Could you check a few things on this model? Use its own coordinates, in mm. A direction names the side the tool comes from. Give positions to 0.01 mm unless a question says otherwise; leave off trailing zeros. Loops run counter-clockwise (first coordinate to the right, second up) from the corner with the lowest first, then second, coordinate; pieces in that order, holes last. Notation, with made-up numbers: M -40,69 L -18,69 A10 ccw -18,75 Z; hole C -6,-14.5 d4. An arc over 180 degrees is marked long. Use a Markdown table: item, result. Add a question column.
1) If I drill on line 1 along Z through (x, y) = (3, 1.65); line 2 along Z through (x, y) = (11.2, 1.5); line 3 along Y through (x, z) = (4.5, 39) (3 decimals), over which ranges is the centre line in solid material (lowest first)? Write a range as [from, to].
2) Suppose I cut it at B-B on y = 0.75. List the corners of the cut face in (x, z) for me (3 decimals).
3) Suppose I cut it at A-A on x = 11.2. List the corners of the cut face in (y, z) for me (3 decimals).
4) Which directions (+Z, -Z, +X, -X, +Y, -Y) give clear straight access to the entire face, cutting with the end or side of a thin tool? Please do faces 4 (the cylindrical face through (1.098, 1.583, 33.354)), 5 (the flat face through (8, 1.905, 30)), 6 (the flat face through (15, 1.905, 30)).
5) Will these pins go through, and if not, where does the flat tip stop? pin 1 Ø0.7 at (x, z) = (1.5, 29) entering from +Y; pin 2 Ø2.5 at (x, z) = (3.5, 33) entering from +Y; pin 3 Ø0.9 at (x, z) = (22, 38) entering from +Y (3 decimals).
6) We'd pull the mould along X, two halves only. Please class faces 1 (the flat face through (20.196, 4.347, 30.128)), 2 (the flat face through (0, 1, 30)), 3 (the flat face through (1, 1.905, 30)): +X half, -X half, draft (parallel to the pull), parting line (faces both ways), or undercut.
```python
from build123d import *

# Parameters (mm, degrees)
SKETCH1_W               = 25.4
SKETCH1_H               = 1.905
BASE_DEPTH              = 61.1124
FINS_DEPTH              = 61.1124
CUT_EXTRUDE1_DEPTH      = 67.365786688
CUT_EXTRUDE1_DEPTH_BACK = 67.365786688
SKETCH3_R               = 1.9939


with BuildPart() as part:
    # Sketch1 → Base (new body)
    with BuildSketch(Plane.XY):
        with Locations((12.7, 0.9525)):
            Rectangle(SKETCH1_W, SKETCH1_H)
    extrude(amount=BASE_DEPTH)

    # Sketch2 → Fins (add)
    with BuildSketch(Plane(origin=(0, 0, 0), x_dir=(-1, 0, 0), z_dir=(0, 0, -1))):
        Polygon((-23.444268018, 1.905), (-25.4, 6.858), (-24.853831982, 6.858), (-22.8981, 1.905), align=None)
        Polygon((-20.040531982, 1.905), (-19.494363964, 1.905), (-20.916831982, 6.858), (-21.463, 6.858), align=None)
        Polygon((-16.979831982, 1.905), (-16.433663964, 1.905), (-16.979831982, 6.858), (-17.526, 6.858), align=None)
        Polygon((-2.794, 1.905), (-2.247831982, 1.905), (0, 6.858), (-0.546168018, 6.858), align=None)
        Polygon((-12.458768018, 6.858), (-11.9126, 6.858), (-12.598263964, 1.905), (-13.144431982, 1.905), align=None)
        Polygon((-8.216968018, 6.858), (-7.6708, 6.858), (-9.245463964, 1.905), (-9.791631982, 1.905), align=None)
        Polygon((-4.483168018, 6.858), (-3.937, 6.858), (-5.943463964, 1.905), (-6.489631982, 1.905), align=None)
    extrude(amount=-FINS_DEPTH)

    # Sketch3 → Cut-Extrude1 (cut, two sides: drawn at the far end of the back side and taken through both)
    with BuildSketch(Plane(origin=(0, 1.905, 0), x_dir=(1, 0, 0), z_dir=(0, 1, 0)).offset(-CUT_EXTRUDE1_DEPTH_BACK)):
        with Locations(Location((11.2, -9.655, 0), (0, 0, 180))):
            Circle(SKETCH3_R)
        with Locations(Location((3, -32.755, 0), (0, 0, 180))):
            Circle(SKETCH3_R)
    extrude(amount=CUT_EXTRUDE1_DEPTH + CUT_EXTRUDE1_DEPTH_BACK, mode=Mode.SUBTRACT)


solid = part.part
```
Answer block:
| question | item | result |
|---|---|---|
| 1 | line 1 | z = [0, 30.76], [34.75, 61.11] |
| 1 | line 2 | z = [0, 7.66], [11.65, 61.11] |
| 1 | line 3 | y = [0, 1.905], [5.468, 6.816] |
| 2 | outline | M 0,0 L 25.4,0 L 25.4,61.112 L 0,61.112 Z; hole C 3,32.755 d3.988; hole C 11.2,9.655 d3.988 |
| 3 | outline | M 0,0 L 1.905,0 L 1.905,7.661 L 0,7.661 Z; M 0,11.649 L 1.905,11.649 L 1.905,61.112 L 0,61.112 Z |
| 4 | face 4 | +Y, -Y |
| 4 | face 5 | +Z, -Z |
| 4 | face 6 | +Z, -Z, +Y |
| 5 | pin 1 | stops at y = 5.53 |
| 5 | pin 2 | passes through |
| 5 | pin 3 | stops at y = 1.905 |
| 6 | face 1 | undercut |
| 6 | face 2 | -X half |
| 6 | face 3 | draft |
